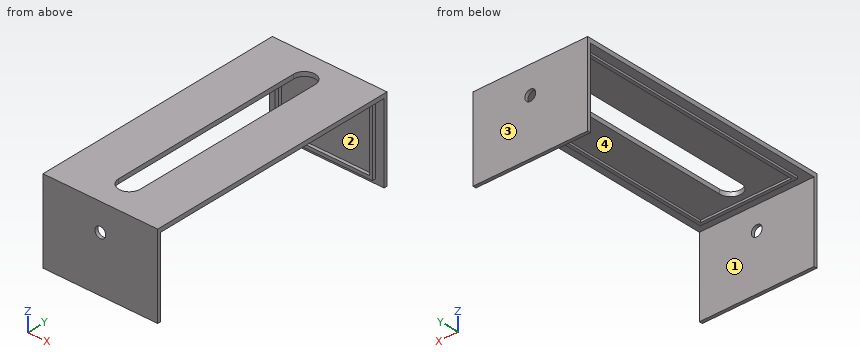
```python
from build123d import *

# Parameters (mm, degrees)
SKETCH1_W           = 90
SKETCH1_H           = 69
SKETCH1_W_2         = 84
SKETCH1_H_2         = 63
BOSS_EXTRUDE1_DEPTH = 3
SKETCH2_W           = 106
SKETCH2_H           = 77
SKETCH2_R           = 5
BOSS_EXTRUDE3_DEPTH = 3
SKETCH3_W           = 230
SKETCH3_H           = 4
BOSS_EXTRUDE4_DEPTH = 106
SKETCH4_W           = 90
SKETCH4_H           = 219
SKETCH4_W_2         = 84
SKETCH4_H_2         = 213
BOSS_EXTRUDE5_DEPTH = 2
SKETCH5_W           = 3
SKETCH5_H           = 77
BOSS_EXTRUDE6_DEPTH = 106
SKETCH6_R           = 5
CUT_EXTRUDE1_DEPTH  = 3
CUT_EXTRUDE2_DEPTH  = 249.270014299


with BuildPart() as part:
    # Sketch1 → Boss-Extrude1 (new body)
    with BuildSketch(Plane(origin=(0, 0, 0), x_dir=(1, 0, 0), z_dir=(0, 1, 0))):
        Rectangle(SKETCH1_W, SKETCH1_H)
        Rectangle(SKETCH1_W_2, SKETCH1_H_2, mode=Mode.SUBTRACT)
    extrude(amount=BOSS_EXTRUDE1_DEPTH)

    # Sketch2 → Boss-Extrude3 (add)
    with BuildSketch(Plane(origin=(0, 3, 0), x_dir=(1, 0, 0), z_dir=(0, 1, 0))):
        Rectangle(SKETCH2_W, SKETCH2_H)
        with Locations(Location((0, -13.15, 0), (0, 0, 270))):
            Circle(SKETCH2_R, mode=Mode.SUBTRACT)
    extrude(amount=BOSS_EXTRUDE3_DEPTH)

    # Sketch3 → Boss-Extrude4 (add)
    with BuildSketch(Plane(origin=(-53, 0, 0), x_dir=(0, -1, 0), z_dir=(-1, 0, 0))):
        with Locations((112, 36.5)):
            Rectangle(SKETCH3_W, SKETCH3_H)
    extrude(amount=-BOSS_EXTRUDE4_DEPTH)

    # Sketch4 → Boss-Extrude5 (add)
    with BuildSketch(Plane(origin=(0, 0, 34.5), x_dir=(1, 0, 0), z_dir=(0, 0, -1))):
        with Locations((0, 109.5)):
            Rectangle(SKETCH4_W, SKETCH4_H)
        with Locations((0, 109.5)):
            Rectangle(SKETCH4_W_2, SKETCH4_H_2, mode=Mode.SUBTRACT)
    extrude(amount=BOSS_EXTRUDE5_DEPTH)

    # Sketch5 → Boss-Extrude6 (add)
    with BuildSketch(Plane(origin=(-53, 0, 0), x_dir=(0, -1, 0), z_dir=(-1, 0, 0))):
        with Locations((228.5, 0)):
            Rectangle(SKETCH5_W, SKETCH5_H)
    extrude(amount=-BOSS_EXTRUDE6_DEPTH)

    # Sketch6 → Cut-Extrude1 (cut)
    with BuildSketch(Plane.XZ.offset(230)):
        with Locations(Location((0, 13.15, 0), (0, 0, 90))):
            Circle(SKETCH6_R)
    extrude(amount=-CUT_EXTRUDE1_DEPTH, mode=Mode.SUBTRACT)

    # Sketch7 → Cut-Extrude2 (cut, through all)
    with BuildSketch(Plane.XY.offset(38.5)):
        with BuildLine():
            Line((10, -20), (10, -200))
            ThreePointArc((10, -200), (0, -210), (-10, -200))
            Line((-10, -200), (-10, -20))
            ThreePointArc((-10, -20), (0, -10), (10, -20))
        make_face()
    extrude(amount=-CUT_EXTRUDE2_DEPTH, mode=Mode.SUBTRACT)


solid = part.part
```
Work out the finished part from the listing and answer in its coordinate system (mm). Face numbers are marked on the shaded views. A direction names the side the tool comes from. Coordinates: 2 decimals unless noted, no trailing zeros. Loops run counter-clockwise (first coordinate to the right, second up) from the corner with the lowest first, then second, coordinate; pieces in that order, holes last.
1) Section B-B (x = 0) is taken. Give the number of separate pieces and of enclosed holes in the cut face, plus the area to 3 significant figures.
Results:
separate pieces: 4
enclosed holes: 0
area: 552 mm2
2) For a pull along X with two mould halves and no side action, classify the marked faces 1 and 2 as +X half, -X half, draft (parallel to the pull), parting line (faces both ways), or undercut.
Results:
face 1: draft
face 2: undercut
3) Section C-C (y = -95) is taken. Give the vertices of the cut face in (x, z), plus the area to 3 significant figures.
Results:
outline: (-53, 34.5) - (-45, 34.5) - (-45, 32.5) - (-42, 32.5) - (-42, 34.5) - (-10, 34.5) - (-10, 38.5) - (-53, 38.5) - close; (10, 34.5) - (42, 34.5) - (42, 32.5) - (45, 32.5) - (45, 34.5) - (53, 34.5) - (53, 38.5) - (10, 38.5) - close
area: 356 mm2
4) Consider probe 1 along Y at (x, z) = (-28, 29.5); probe 2 along X at (y, z) = (-228.4, 13.15); probe 3 along Z at (x, y) = (-44, -106). Determine where each line is inside the solid, lowest interval first.
Results:
probe 1: y = -230 to -227, 3 to 6
probe 2: x = -53 to -5, 5 to 53
probe 3: z = 32.5 to 38.5
5) Flat-ended cylindrical pins translate along their axes: pin 1 (25 mm diameter, centred on x = 17.5, y = -97.5, fed in from -Z); pin 2 (2 mm diameter, centred on y = -110.5, z = 33, fed in from -X); pin 3 (1.5 mm diameter, centred on x = -6, y = 1.5, fed in from -Z). Find the tip coordinate at first contact, or state that the pin passes through.
Results:
pin 1: stops at z = 34.5
pin 2: stops at x = -45
pin 3: stops at z = -34.5
6) Section D-D (z = -13) is taken. Give the vertices of the cut face in (x, y).
Results:
outline: (-53, -230) - (53, -230) - (53, -227) - (-53, -227) - close; (-53, 3) - (-45, 3) - (-45, 0) - (-42, 0) - (-42, 3) - (42, 3) - (42, 0) - (45, 0) - (45, 3) - (53, 3) - (53, 6) - (-53, 6) - close
7) For the marked faces 3 and 4, determine the directions among +Z, -Z, +X, -X, +Y, -Y from which every point of the face is accessible in a straight line to the end or side of a thin tool.
Results:
face 3: +Z, -Z, +X, -X, +Y
face 4: -Z
8) Section A-A (z = 13.15) is taken. Give the vertices of the cut face in (x, y), plus the area to 3 significant figures.
Results:
outline: (-53, -230) - (-5, -230) - (-5, -227) - (-53, -227) - close; (-53, 3) - (-45, 3) - (-45, 0) - (-42, 0) - (-42, 3) - (-5, 3) - (-5, 6) - (-53, 6) - close; (5, -230) - (53, -230) - (53, -227) - (5, -227) - close; (5, 3) - (42, 3) - (42, 0) - (45, 0) - (45, 3) - (53, 3) - (53, 6) - (5, 6) - close
area: 594 mm2
